Could you check a few things on this model? Use its own coordinates, in mm. A direction names the side the tool comes from. Coordinates: 2 decimals unless noted, no trailing zeros. Order: outer loops, then holes, each group sorted by start corner. A loop starts at its lowest first (then second) coordinate and runs counter-clockwise, first axis right, second up.
```python
from build123d import *

# Parameters (mm, degrees)
F0_W      = 23.2918
F0_H      = 10.1092
F1_DEPTH  = 0.7366
F3_DEPTH  = 25.4
F4_R      = 1.2827
F4_R_2    = 3.3782
F5_DEPTH  = 0.7376
F6_R      = 0.6985
F7_DEPTH  = 0.7366
F9_DEPTH  = 2.1844
F10_W     = 1.4986
F10_H     = 1.9812
F11_DEPTH = 18.0604
F12_W     = 1.4986
F12_H     = 1.9812
F13_DEPTH = 18.0604
F15_DEPTH = 0.6858
F17_DEPTH = 0.6858


with BuildPart() as f1:
    # F0 (on Front) → F1 (new body)
    with BuildSketch(Plane.XZ):
        Rectangle(F0_W, F0_H)
    extrude(amount=F1_DEPTH)

    # F2 (on face) → F3 (cut)
    with BuildSketch(Plane.XZ.offset(0.7366)):
        with BuildLine():
            Line((-10.3464885777, 2.4295455305), (-6.4135, 5.0546))
            Line((-6.4135, 5.0546), (-11.6459, 5.0546))
            Line((-11.6459, 5.0546), (-11.6459, 0))
            ThreePointArc((-11.6459, 0), (-11.3006427313, 1.3776031295), (-10.3464885777, 2.4295455305))
        make_face()
        with BuildLine():
            Line((-11.6459, -5.0546), (-6.4135, -5.0546))
            Line((-6.4135, -5.0546), (-10.3464885777, -2.4295455305))
            ThreePointArc((-10.3464885777, -2.4295455305), (-11.3006427313, -1.3776031295), (-11.6459, 0))
            Line((-11.6459, 0), (-11.6459, -5.0546))
        make_face()
        with BuildLine():
            ThreePointArc((11.6459, 0), (11.3006427313, -1.3776031295), (10.3464885777, -2.4295455305))
            Line((10.3464885777, -2.4295455305), (6.4135, -5.0546))
            Line((6.4135, -5.0546), (11.6459, -5.0546))
            Line((11.6459, -5.0546), (11.6459, 0))
        make_face()
        with BuildLine():
            ThreePointArc((10.3464885777, 2.4295455305), (11.3006427313, 1.3776031295), (11.6459, 0))
            Line((11.6459, 0), (11.6459, 5.0546))
            Line((11.6459, 5.0546), (6.4135, 5.0546))
            Line((6.4135, 5.0546), (10.3464885777, 2.4295455305))
        make_face()
    extrude(amount=-F3_DEPTH, mode=Mode.SUBTRACT)

    # F4 (on face) → F5 (cut, through all)
    with BuildSketch(Plane.XZ.offset(0.7366)):
        with Locations((-8.7249, 0)):
            Circle(F4_R)
        Circle(F4_R_2)
        with Locations((8.7249, 0)):
            Circle(F4_R)
    extrude(amount=-F5_DEPTH, mode=Mode.SUBTRACT)

    # F6 (on face) → F7 (join)
    with BuildSketch(Plane.XZ.offset(0.7366)):
        with BuildLine():
            ThreePointArc((-4.6482, 0), (-5.3467, 0.6985), (-6.0452, 0))
            ThreePointArc((-6.0452, 0), (-5.3467, -0.6985), (-4.6482, 0))
        make_face()
        with Locations((5.3467, 0)):
            Circle(F6_R)
    extrude(amount=F7_DEPTH)

    # F8 (on face) → F9 (join)
    with BuildSketch(Plane.XZ.offset(0.7366)):
        with BuildLine():
            Line((-6.4135, 2.3876), (-2.3898957048, 2.3876))
            ThreePointArc((-2.3898957048, 2.3876), (0, 3.3782), (2.3898957048, 2.3876))
            Line((2.3898957048, 2.3876), (6.4135, 2.3876))
            Line((6.4135, 2.3876), (6.4135, 5.0546))
            Line((6.4135, 5.0546), (-6.4135, 5.0546))
            Line((-6.4135, 5.0546), (-6.4135, 2.3876))
        make_face()
        with BuildLine():
            Line((-6.4135, -2.3876), (-6.4135, -5.0546))
            Line((-6.4135, -5.0546), (6.4135, -5.0546))
            Line((6.4135, -5.0546), (6.4135, -2.3876))
            Line((6.4135, -2.3876), (2.3898957048, -2.3876))
            ThreePointArc((2.3898957048, -2.3876), (0, -3.3782), (-2.3898957048, -2.3876))
            Line((-2.3898957048, -2.3876), (-6.4135, -2.3876))
        make_face()
    extrude(amount=F9_DEPTH)

    # F10 (on face) → F11 (cut, through all)
    with BuildSketch(Plane(origin=(-6.4135, 0, 0), x_dir=(0, -1, 0), z_dir=(-1, 0, 0))):
        with Locations((1.4859, 3.3782)):
            Rectangle(F10_W, F10_H)
    extrude(amount=-F11_DEPTH, mode=Mode.SUBTRACT)

    # F12 (on face) → F13 (cut, through all)
    with BuildSketch(Plane(origin=(-6.4135, 0, 0), x_dir=(0, -1, 0), z_dir=(-1, 0, 0))):
        with Locations((1.4859, -3.3782)):
            Rectangle(F12_W, F12_H)
    extrude(amount=-F13_DEPTH, mode=Mode.SUBTRACT)

    # F14 (on face) → F15 (cut)
    with BuildSketch(Plane.XZ.offset(2.921)):
        with BuildLine():
            Line((2.3898957048, 2.3876), (3.8692296132, 2.3876))
            ThreePointArc((3.8692296132, 2.3876), (0, 4.5466), (-3.8692296132, 2.3876))
            Line((-3.8692296132, 2.3876), (-2.3898957048, 2.3876))
            ThreePointArc((-2.3898957048, 2.3876), (0, 3.3782), (2.3898957048, 2.3876))
        make_face()
    extrude(amount=-F15_DEPTH, mode=Mode.SUBTRACT)

    # F16 (on face) → F17 (cut)
    with BuildSketch(Plane.XZ.offset(2.921)):
        with BuildLine():
            Line((-2.3898957048, -2.3876), (-3.8692296132, -2.3876))
            ThreePointArc((-3.8692296132, -2.3876), (0, -4.5466), (3.8692296132, -2.3876))
            Line((3.8692296132, -2.3876), (2.3898957048, -2.3876))
            ThreePointArc((2.3898957048, -2.3876), (0, -3.3782), (-2.3898957048, -2.3876))
        make_face()
    extrude(amount=-F17_DEPTH, mode=Mode.SUBTRACT)


solid = f1.part
```
Item 1: For pin 1 Ø1.1 at (y, z) = (-1.5, -4) entering from +X; pin 2 Ø4 at (x, z) = (0, 0) entering from -Y; pin 3 Ø1.5 at (y, z) = (-1, 1.5) entering from -X, each with a flat end and sliding along its axis, tell me the tip position at first contact or that it passes through.
Item 2: Suppose I cut it at B-B (y = -1.2). List the corners of the cut face in (x, z) for me, and give its area (3 significant figures).
Item 3: Thinking about a two-plate mould opening in Y: for faces 5 (the face through (-3, 0, 2)), 6 (the face through (6.414, -2.5, 4)), 7 (the face through (0, -1, -4.369)), which applies, +Y half, -Y half, draft (parallel to the pull), parting line (faces both ways), or undercut?
Item 4: Suppose I cut it at D-D (z = -1). List the corners of the cut face in (x, y) for me, and give its area (3 significant figures).
Item 5: Suppose I cut it at A-A (x = 0). List the corners of the cut face in (y, z) for me, and give its area (3 significant figures).
Item 6: I need wall thicknesses on line 1 (Z direction, x = 0, y = -0.5); line 2 (Y direction, x = -6, z = 3.5); line 3 (Z direction, x = -4.5, y = -2.6). Which ranges of each line are inside material? Lowest first, please.
Item 7: Suppose I cut it at C-C (z = 3.75). List the corners of the cut face in (x, y) for me.
Item 8: Which directions (+Z, -Z, +X, -X, +Y, -Y) give clear straight access to the entire face, cutting with the end or side of a thin tool? Please do faces 1 (the face through (-5, -1.473, 0)), 2 (the face through (6.414, -2.5, -4)), 3 (the face through (-6.414, -2.5, 4)), 4 (the face through (-0.065, -2.583, -4.546)).
Geometry results:
1. pin 1: stops at x = 6.41
1. pin 2: passes through
1. pin 3: stops at x = -11.53
2. outline: (-6.41, -5.05) - (6.41, -5.05) - (6.41, -4.37) - (-6.41, -4.37) - close; (-6.41, 4.37) - (6.41, 4.37) - (6.41, 5.05) - (-6.41, 5.05) - close; circle Ø1.4 at (-5.35, 0); circle Ø1.4 at (5.35, 0)
2. area: 20.7 mm2
3. face 5: +Y half
3. face 6: draft
3. face 7: undercut
4. outline: (-11.47, -0.74) - (-9.53, -0.74) - (-9.53, 0) - (-11.47, 0) - close; (-7.92, -0.74) - (-3.23, -0.74) - (-3.23, 0) - (-7.92, 0) - close; (3.23, -0.74) - (7.92, -0.74) - (7.92, 0) - (3.23, 0) - close; (9.53, -0.74) - (11.47, -0.74) - (11.47, 0) - (9.53, 0) - close
4. area: 9.78 mm2
5. outline: (-2.92, -5.05) - (0, -5.05) - (0, -3.38) - (-0.74, -3.38) - (-0.74, -4.37) - (-2.24, -4.37) - (-2.24, -4.55) - (-2.92, -4.55) - close; (-2.92, 4.55) - (-2.24, 4.55) - (-2.24, 4.37) - (-0.74, 4.37) - (-0.74, 3.38) - (0, 3.38) - (0, 5.05) - (-2.92, 5.05) - close
5. area: 5.22 mm2
6. line 1: z = -5.05 to -3.38, 3.38 to 5.05
6. line 2: y = -2.92 to -2.24, -0.74 to 0
6. line 3: z = -5.05 to -2.39, 2.39 to 5.05
7. outline: (-8.37, -0.74) - (8.37, -0.74) - (8.37, 0) - (-8.37, 0) - close; (-6.41, -2.92) - (-2.57, -2.92) - (-2.57, -2.24) - (-6.41, -2.24) - close; (2.57, -2.92) - (6.41, -2.92) - (6.41, -2.24) - (2.57, -2.24) - close
8. face 1: +X, -X, -Y
8. face 2: +Z, -Z, +X, -Y
8. face 3: +Z, -Z, -X, -Y
8. face 4: -Y
